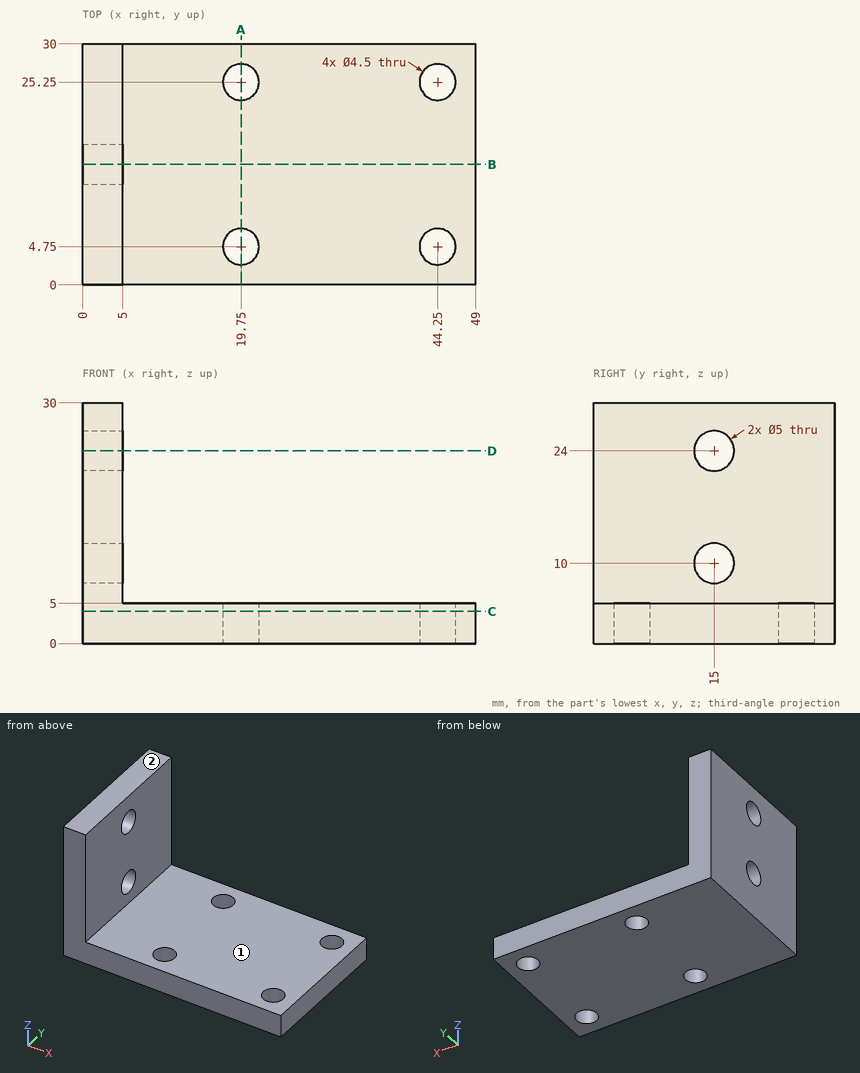
Geometry: see drawing. Coordinates: mm, zero at the bounding-box minimum. A direction names the side the tool comes from. Coordinates: 2 decimals unless noted, no trailing zeros. Loops run counter-clockwise (first coordinate to the right, second up) from the corner with the lowest first, then second, coordinate; pieces in that order, holes last. Notation, with made-up numbers: M -13.75,-38.75 L 8.25,-38.75 A12 ccw 8.25,-33.75 Z; hole C 12,83 d4. An arc over 180 degrees is marked long. Answer in a Markdown table with one row per item.
Q1. First-contact query: pin 1 (3 mm diameter, centred on x = 29.5, z = 5.5, fed in from -Y); pin 2 (4 mm diameter, centred on y = 15, z = 10, fed in from +X); pin 3 (6 mm diameter, centred on y = 12, z = 9.5, fed in from +X); pin 4 (1 mm diameter, centred on x = 21.5, y = 16.5, fed in from +Z). Flat tips, straight axial feed; report the tip coordinate or a pass-through.
Answers below:
| item | result |
|---|---|
| pin 1 | stops at y = 0 |
| pin 2 | passes through |
| pin 3 | stops at x = 5 |
| pin 4 | stops at z = 5 |
Q2. Section C-C on z = 4. Return the cut outline in (x, y), plus the area to 3 significant figures.
Answers below:
| item | result |
|---|---|
| outline | M 0,0 L 49,0 L 49,30 L 0,30 Z; hole C 19.75,4.75 d4.5; hole C 19.75,25.25 d4.5; hole C 44.25,4.75 d4.5; hole C 44.25,25.25 d4.5 |
| area | 1,410 mm^2 |
Q3. Section D-D on z = 24. Return the cut outline in (x, y), plus the area to 3 significant figures.
Answers below:
| item | result |
|---|---|
| outline | M 0,0 L 5,0 L 5,12.5 L 0,12.5 Z; M 0,17.5 L 5,17.5 L 5,30 L 0,30 Z |
| area | 125 mm^2 |
Q4. Section B-B on y = 15. Return the cut outline in (x, z).
Answers below:
| item | result |
|---|---|
| outline | M 0,0 L 49,0 L 49,5 L 5,5 L 5,7.5 L 0,7.5 Z; M 0,12.5 L 5,12.5 L 5,21.5 L 0,21.5 Z; M 0,26.5 L 5,26.5 L 5,30 L 0,30 Z |
Q5. Ray query, probe 1 along Y at (x, z) = (44.25, 3.3); probe 2 along Y at (x, z) = (2.95, 10); probe 3 along Z at (x, y) = (21.5, 10). Return the intervals inside material, ascending. Write a range as from..to.
Answers below:
| item | result |
|---|---|
| probe 1 | y = 0..2.5, 7..23, 27.5..30 |
| probe 2 | y = 0..12.5, 17.5..30 |
| probe 3 | z = 0..5 |
Q6. Set-up query: the marked faces 1 and 2. Return all of +Z, -Z, +X, -X, +Y, -Y with unobstructed straight access to the full face (end or side cutting, diameter ignored); none if empty.
Answers below:
| item | result |
|---|---|
| face 1 | +Z, +X, +Y, -Y |
| face 2 | +Z, +X, -X, +Y, -Y |
Q7. Section A-A on x = 19.75. Return the cut outline in (y, z).
Answers below:
| item | result |
|---|---|
| outline | M 0,0 L 2.5,0 L 2.5,5 L 0,5 Z; M 7,0 L 23,0 L 23,5 L 7,5 Z; M 27.5,0 L 30,0 L 30,5 L 27.5,5 Z |
